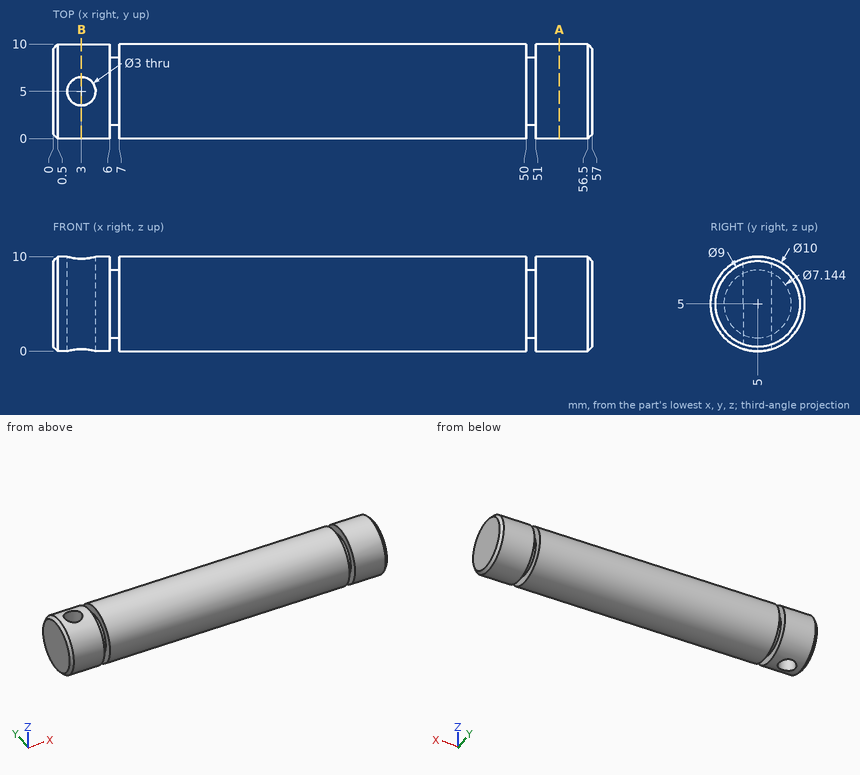
Geometry: see drawing. Coordinates: mm, zero at the bounding-box minimum. Round coordinates to 2 decimals unless told otherwise and drop trailing zeros. Loops run counter-clockwise (first coordinate to the right, second up) from the corner with the lowest first, then second, coordinate; pieces in that order, holes last. Notation, with made-up numbers: (67, 70.25) - (121, 70.25) arc R12 cw to (121, 92.25) - close; hole circle Ø9 at (-7, 85.5). An arc over 180 degrees is marked (long way). Write item = value, one per line. Start each with the question number.
(1) Pin query (flat end, axial travel): pin 1 (5 mm diameter, centred on x = 22.5, y = 7, fed in from +Z); pin 2 (1 mm diameter, centred on x = 36.5, y = 7, fed in from -Z); pin 3 (1.5 mm diameter, centred on x = 6.5, z = 2, fed in from -Y). Return the tip coordinate at first contact, or that it passes through.
(2) Section query B-B, the plane x = 3. Output: boundary loops of the cut face in (y, z), plus the area to 3 significant figures.
(3) Section query A-A, the plane x = 53.5. Output: boundary loops of the cut face in (y, z).
(4) Ray query, line 1 along X through (y, z) = (5, 7.75); line 2 along X through (y, z) = (8.5, 7.75); line 3 along Y through (x, z) = (3, 1.5). Return the intervals inside material, ascending. Write a range as from..to.
Conclusion:
q1.pin_1 = 10
q1.pin_2 = 0.23
q1.pin_3 = 0.64
q2.outline = (3.5, 0.23) - (3.5, 9.77) arc R5 ccw to start; (6.5, 0.23) arc R5 ccw to (6.5, 9.77) - close
q2.area = 49.0 mm2
q3.outline = circle Ø10 at (5, 5)
q4.line_1 = 0..1.5, 4.5..57
q4.line_2 = 0..6, 7..50, 51..57
q4.line_3 = 1.43..3.5, 6.5..8.57
